For this review, take the finished solid that the model builds, in its own axes (mm). Round coordinates to 2 decimals unless told otherwise and drop trailing zeros. Write each loop counter-clockwise with the first axis right and the second up, starting at its lowest first coordinate (ties: lowest second). Pieces come first, ordered by that corner, then holes. Notation, with made-up numbers: (57.5, 68) -> (101.5, 68) arc R29 ccw to (101.5, 95) -> close; hole circle Ø9 at (86, -6.5). An arc over 180 degrees is marked (long way). Answer as CSV lines item,"result". Start each with the question number.
Item 1: Mouldability with a two-part tool opening along Z and no side actions: class faces 1 (the flat face through (221.107, 6.439, 200.355)), 2 (the flat face through (113, 5, 406.4)), 3 (the flat face through (146, 6.35, 203)) as +Z half, -Z half, draft (parallel to the pull), parting line (faces both ways), or undercut.
Item 2: Wall thickness on probe 1 along X at (y, z) = (10.25, 105.5); probe 2 along Z at (x, y) = (198, 9.5); probe 3 along Z at (x, y) = (46, 10.75): over which ranges is each line inside the solid? List them lowest first. Write a range as from..to.
Item 3: For pin 1 Ø1.5 at (x, y) = (170.5, 4.5) entering from -Z; pin 2 Ø4 at (x, z) = (143, 205.5) entering from +Y; pin 3 Ø1.9 at (x, y) = (82, 10.5) entering from -Z; pin 4 Ø1.9 at (y, z) = (11, 205) entering from +X, all flat-tipped, find the tip position at first contact; note any pin that passes through.
Item 4: Take a section at A-A on x = 157. Give the boundary of the cut face in (y, z), then the cut area to 3 significant figures.
```python
from build123d import *

# Parameters (mm, degrees)
BOSS_EXTRUDE1_DEPTH = 406.4
SKETCH2_W           = 223.774
SKETCH2_H           = 6.35
CUT_EXTRUDE1_DEPTH  = 2.3622
CAVITY1_START       = 196.85
CAVITY1_OUTLINE_W   = 86.97620095
CAVITY1_OUTLINE_H   = 6.35
CAVITY1_DEPTH       = 12.7
SKETCH3_W           = 266.782886341
SKETCH3_H           = 6.35
CUT_EXTRUDE2_DEPTH  = 6.35


# Read off the part's stored shape, not the designer's step: Cavity1
with BuildPart() as part:
    # Sketch1 → Boss-Extrude1 (new body)
    with BuildSketch(Plane.XY):
        Polygon((0, 0), (0, 12.7), (218.513487758, 12.7), (223.774, 0), align=None)
    extrude(amount=BOSS_EXTRUDE1_DEPTH)

    # Sketch2 → Cut-Extrude1 (cut)
    with BuildSketch(Plane.XZ.offset(-12.7)):
        with Locations((111.887, 403.225)):
            Rectangle(SKETCH2_W, SKETCH2_H)
    extrude(amount=CUT_EXTRUDE1_DEPTH, mode=Mode.SUBTRACT)

    # Cavity1 outline → Cavity1 (cut)
    with BuildSketch(Plane.XY.offset(CAVITY1_START)):
        with Locations((146.563552259, 9.525)):
            Rectangle(CAVITY1_OUTLINE_W, CAVITY1_OUTLINE_H)
    extrude(amount=CAVITY1_DEPTH, mode=Mode.SUBTRACT)

    # Sketch3 → Cut-Extrude2 (cut)
    with BuildSketch(Plane(origin=(0, 12.7, 0), x_dir=(1, 0, 0), z_dir=(0, 1, 0))):
        with Locations((133.39144317, -3.175)):
            Rectangle(SKETCH3_W, SKETCH3_H)
    extrude(amount=-CUT_EXTRUDE2_DEPTH, mode=Mode.SUBTRACT)


solid = part.part
```
Output values:
1,face 1,"draft"
1,face 2,"+Z half"
1,face 3,"undercut"
2,probe 1,"x = 0..219.53"
2,probe 2,"z = 6.35..406.4"
2,probe 3,"z = 6.35..400.05"
3,pin 1,"stops at z = 0"
3,pin 2,"stops at y = 6.35"
3,pin 3,"stops at z = 6.35"
3,pin 4,"stops at x = 219.61"
4,outline,"(0, 0) -> (6.35, 0) -> (6.35, 6.35) -> (12.7, 6.35) -> (12.7, 196.85) -> (6.35, 196.85) -> (6.35, 209.55) -> (12.7, 209.55) -> (12.7, 400.05) -> (10.34, 400.05) -> (10.34, 406.4) -> (0, 406.4) -> close"
4,area,"5,030 mm^2"
